from build123d import *

# Parameters (mm, degrees)
F1_DEPTH = 20


with BuildPart() as f1:
    # F0 (on Front) → F1 (new body)
    with BuildSketch(Plane.XZ):
        with BuildLine():
            ThreePointArc((670.6236231078, 66.3387719466), (309.6652800425, 79.699666295), (-51.2863881664, 66.159646229))
            ThreePointArc((-51.2863881664, 66.159646229), (-7.9443574248, 44.95304923), (9.5906005169, 0))
            Line((9.5906005169, 0), (606.8129005169, 0))
            ThreePointArc((606.8129005169, 0), (625.3549203284, 46.0234749366), (670.6236231078, 66.3387719466))
        make_face()
        with BuildLine():
            ThreePointArc((9.5906005169, 0), (-11.5233416669, -48.5557630622), (-61.4352457375, -66.2267141723))
            ThreePointArc((-61.4352457375, -66.2267141723), (306.2183279395, -80.2613301697), (673.8779251557, -66.3854064699))
            ThreePointArc((673.8779251557, -66.3854064699), (626.4974201628, -47.1824642266), (606.8129005169, 0))
            Line((606.8129005169, 0), (9.5906005169, 0))
        make_face()
        with BuildLine():
            ThreePointArc((-51.2863881664, 66.159646229), (-61.8356743177, 65.3581420921), (-72.3831869864, 64.5336278799))
            ThreePointArc((-72.3831869864, 64.5336278799), (-122.9890910705, -5.1236602419), (-62.2662803124, -66.1632831952))
            ThreePointArc((-62.2662803124, -66.1632831952), (-61.8507643875, -66.195016535), (-61.4352457375, -66.2267141723))
            ThreePointArc((-61.4352457375, -66.2267141723), (-11.5233416669, -48.5557630622), (9.5906005169, 0))
            ThreePointArc((9.5906005169, 0), (-7.9443574248, 44.95304923), (-51.2863881664, 66.159646229))
        make_face()
        with BuildLine():
            ThreePointArc((685.7701519609, 65.1883017839), (678.1973379425, 65.7694667188), (670.6236231078, 66.3387719466))
            ThreePointArc((670.6236231078, 66.3387719466), (625.3549203284, 46.0234749366), (606.8129005169, 0))
            ThreePointArc((606.8129005169, 0), (626.4974201628, -47.1824642266), (673.8779251557, -66.3854064699))
            ThreePointArc((673.8779251557, -66.3854064699), (678.2691787155, -66.0505126994), (682.6601263672, -65.7116316233))
            ThreePointArc((682.6601263672, -65.7116316233), (723.3784886527, -43.4715349899), (739.5906005169, 0))
            ThreePointArc((739.5906005169, 0), (724.3968729532, 42.2674679045), (685.7701519609, 65.1883017839))
        make_face()
    extrude(amount=F1_DEPTH)


solid = f1.part
Can you work these out from the model? Positions are in its coordinate system, mm. Round coordinates to 2 decimals unless told otherwise and drop trailing zeros. Order: outer loops, then holes, each group sorted by start corner. A loop starts at its lowest first (then second) coordinate and runs counter-clockwise, first axis right, second up. Notation, with made-up numbers: (-27.75, -22) -> (11.25, -22) arc R18 cw to (11.25, -8) -> close; hole circle Ø1 at (-37, 65). An arc over 180 degrees is marked (long way). Write each question's results on one line, items separated by ' | '. Start each with the question number.
Item 1: If we section it at A-A, the plane y = -4.5: Write out the boundary of the cut face in (x, z).
Item 2: Please list where these lines run through material, in increasing order: L1, parallel to Z at x = 315, y = -5.5; L2, parallel to Z at x = 424.5, y = -3.5; L3, parallel to X at y = -17.25, z = 38.
Item 3: If we section it at B-B, the plane x = 0: Write out the boundary of the cut face in (y, z), then the cut area to 3 significant figures.
Item 4: If we section it at C-C, the plane z = 35: Write out the boundary of the cut face in (x, y).
Item 5: Will these pins go through, and if not, where does the flat tip stop? pin 1 (1.5 mm diameter, centred on y = -14.5, z = -7, fed in from -X); pin 2 (5 mm diameter, centred on y = -13.5, z = 21, fed in from +X); pin 3 (8 mm diameter, centred on y = -9.5, z = -8, fed in from -X).
Results:
1) outline: (-72.38, 64.53) arc R66.39 ccw to (-62.27, -66.16) arc R4849.99 ccw to (-61.44, -66.23) arc R4850 ccw to (673.88, -66.39) arc R4850 ccw to (682.66, -65.71) arc R66.39 ccw to (685.77, 65.19) arc R4850 ccw to (670.62, 66.34) arc R4850 ccw to (-51.29, 66.16) arc R4850 ccw to start
2) L1: z = -80.26 to 79.7 | L2: z = -78.84 to 78.37 | L3: x = -111.24 to 727.64
3) outline: (-20, -70.52) -> (0, -70.52) -> (0, 69.73) -> (-20, 69.73) -> close | area: 2,800 mm2
4) outline: (-113.21, -20) -> (729.62, -20) -> (729.62, 0) -> (-113.21, 0) -> close
5) pin 1: stops at x = -122.89 | pin 2: stops at x = 736.96 | pin 3: stops at x = -123.07
